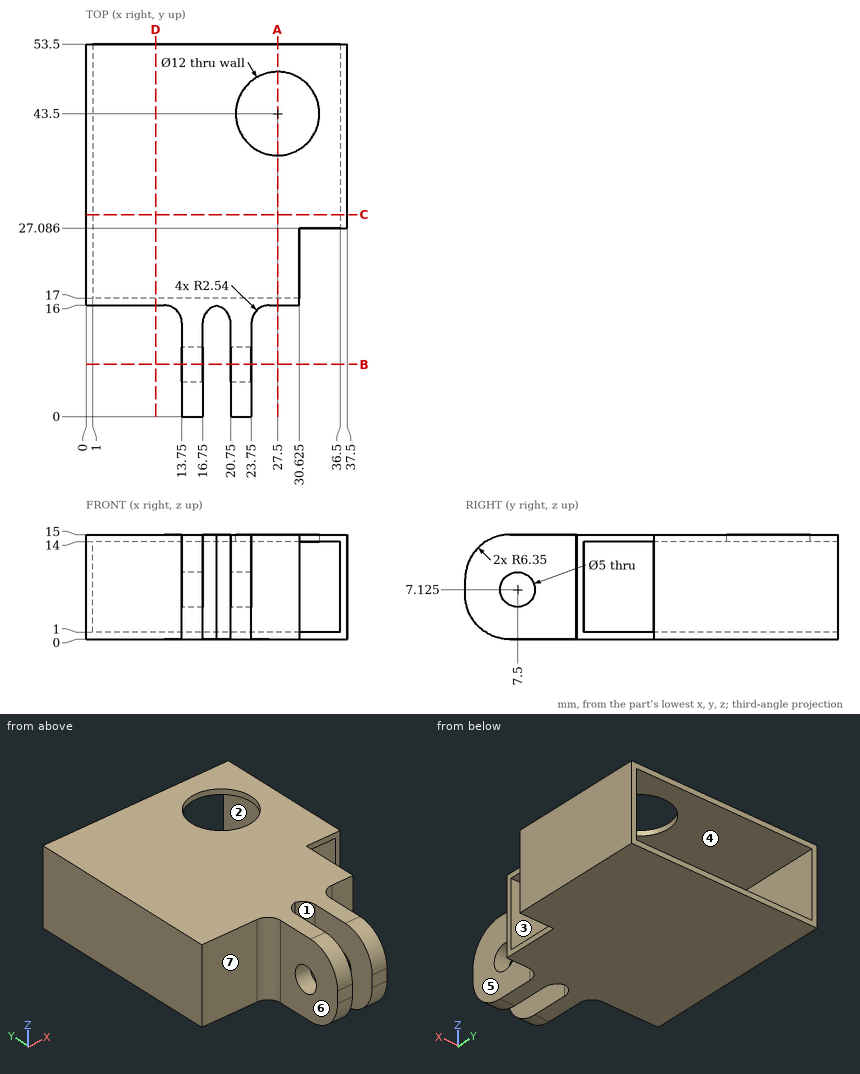
Answer from the drawing. Dimensions are ordinates in mm from the lowest x, y and z of the part. A direction names the side the tool comes from. Coordinates: 2 decimals unless noted, no trailing zeros. Write each loop counter-clockwise with the first axis right and the second up, starting at its lowest first coordinate (ties: lowest second). Pieces come first, ordered by that corner, then holes. Notation, with made-up numbers: M 88,76.25 L 144,76.25 A16 ccw 144,89.25 Z; hole C 65,67 d5. An arc over 180 degrees is marked long. Put each result on its own line as item: value. Start each with the question number.
1. A cutting plane is placed at A-A on x = 27.5. Write down the section's boundary in (y, z).
2. Which of the six approach directions +Z, -Z, +X, -X, +Y, -Y give full straight-line access (tool end or side, diameter ignored) to the marked faces 1, 2 and 3?
3. Flat-ended cylindrical pins translate along their axes: P1, Ø6.5, axis at y = 9.5, z = 7, coming from the +X side; P2, Ø3, axis at y = 16, z = 7.5, coming from the +X side (3 decimals); P3, Ø6.5, axis at x = 17.5, z = 5, coming from the +Y side; P4, Ø3.5, axis at x = 33.5, z = 6, coming from the -Y side. Find the tip coordinate at first contact, or state that the pin passes through.
4. A cutting plane is placed at C-C on y = 29. Write down the section's boundary in (x, z), then the cut area to 3 significant figures.
5. For a pull along X with two mould halves and no side action, classify the marked faces 4, 5, 6 and 7 as pulls with the +X half, pulls with the -X half, needs draft (parallel to the pull), parting line crosses it, or undercut.
6. A cutting plane is placed at B-B on y = 7.5. Write down the section's boundary in (x, z) (3 decimals), then the cut area to 3 significant figures.
7. Consider line 1 (Z direction, x = 20.5, y = 29); line 2 (Z direction, x = 15.9, y = 7.5) (3 decimals); line 3 (X direction, y = 37, z = 8.25). Determine where each line is inside the solid, lowest interval first. Write a range as from..to.
8. A cutting plane is placed at D-D on x = 10. Write down the section's boundary in (y, z).
Resolved:
1. outline: M 16,0 L 53.5,0 L 53.5,1 L 17,1 L 17,14 L 37.5,14 L 37.5,15 L 16,15 Z; M 49.5,14 L 53.5,14 L 53.5,15 L 49.5,15 Z
2. face 1: +Z, -Z, -Y
2. face 2: +Y, -Y
2. face 3: +X, +Y
3. P1: stops at x = 23.75
3. P2: stops at x = 30.625
3. P3: stops at y = 17
3. P4: passes through
4. outline: M 0,0 L 37.5,0 L 37.5,15 L 0,15 Z; hole M 1,1 L 36.5,1 L 36.5,14 L 1,14 Z
4. area: 101 mm2
5. face 4: undercut
5. face 5: pulls with the +X half
5. face 6: pulls with the -X half
5. face 7: needs draft
6. outline: M 13.75,0 L 16.75,0 L 16.75,4.625 L 13.75,4.625 Z; M 13.75,9.625 L 16.75,9.625 L 16.75,15 L 13.75,15 Z; M 20.75,0 L 23.75,0 L 23.75,4.625 L 20.75,4.625 Z; M 20.75,9.625 L 23.75,9.625 L 23.75,15 L 20.75,15 Z
6. area: 60.0 mm2
7. line 1: z = 0..1, 14..15
7. line 2: z = 0..4.625, 9.625..15
7. line 3: x = 0..1, 36.5..37.5
8. outline: M 16,0 L 53.5,0 L 53.5,1 L 17,1 L 17,14 L 53.5,14 L 53.5,15 L 16,15 Z
